Can you work these out from the model? Positions are in its coordinate system, mm. A direction names the side the tool comes from. Round coordinates to 2 decimals unless told otherwise and drop trailing zeros. Order: outer loops, then holes, each group sorted by start corner. A loop starts at its lowest first (then second) coordinate and runs counter-clockwise, first axis right, second up. Notation, with made-up numbers: (62.5, 50) -> (85.5, 50) arc R14 ccw to (85.5, 59) -> close; hole circle Ø9 at (-24, 54). An arc over 180 degrees is marked (long way). One line per item, written item: value.
```python
from build123d import *

# Parameters (mm, degrees)
EXTRUDE001_DEPTH = 3
EXTRUDE_DEPTH    = 5
PAD_DEPTH        = 6


with BuildPart() as extrude001:
    # RegularPolygon001 → Extrude001 (new body)
    with BuildSketch(Plane(origin=(0, 0, -2), x_dir=(0, 1, 0), z_dir=(0, 0, 1))):
        Polygon((0, -2.31), (2.000519, -1.155), (2.000519, 1.155), (0, 2.31), (-2.000519, 1.155), (-2.000519, -1.155), align=None)
    extrude(amount=-EXTRUDE001_DEPTH)


with BuildPart() as extrude_body:
    # RegularPolygon → Extrude (new body)
    with BuildSketch(Plane(origin=(0, 0, 0), x_dir=(0, 1, 0), z_dir=(0, 0, 1))):
        Polygon((0, -4.85), (4.200223, -2.425), (4.200223, 2.425), (0, 4.85), (-4.200223, 2.425), (-4.200223, -2.425), align=None)
    extrude(amount=-EXTRUDE_DEPTH)


with BuildPart() as fusion:
    # Sketch → Pad (new body)
    with BuildSketch(Plane.XY):
        with BuildLine():
            ThreePointArc((1.737208, 7.038793), (0, 9), (-1.737208, 7.038793))
            ThreePointArc((-3.748787, 6.20557), (-2.356657, 5.689474), (-1.737208, 7.038793))
            ThreePointArc((-3.748787, 6.20557), (-6.363961, 6.363961), (-6.20557, 3.748787))
            ThreePointArc((-7.038793, 1.737208), (-5.689474, 2.356657), (-6.20557, 3.748787))
            ThreePointArc((-7.038793, 1.737208), (-9, 0), (-7.038793, -1.737208))
            ThreePointArc((-6.20557, -3.748787), (-5.689474, -2.356657), (-7.038793, -1.737208))
            ThreePointArc((-6.20557, -3.748787), (-6.363961, -6.363961), (-3.748787, -6.20557))
            ThreePointArc((-1.737208, -7.038793), (-2.356657, -5.689474), (-3.748787, -6.20557))
            ThreePointArc((-1.737208, -7.038793), (0, -9), (1.737208, -7.038793))
            ThreePointArc((3.748787, -6.20557), (2.356657, -5.689474), (1.737208, -7.038793))
            ThreePointArc((3.748787, -6.20557), (6.363961, -6.363961), (6.20557, -3.748787))
            ThreePointArc((7.038793, -1.737208), (5.689474, -2.356657), (6.20557, -3.748787))
            ThreePointArc((7.038793, -1.737208), (9, 0), (7.038793, 1.737208))
            ThreePointArc((6.20557, 3.748787), (5.689474, 2.356657), (7.038793, 1.737208))
            ThreePointArc((6.20557, 3.748787), (6.363961, 6.363961), (3.748787, 6.20557))
            ThreePointArc((1.737208, 7.038793), (2.356657, 5.689474), (3.748787, 6.20557))
        make_face()
    extrude(amount=-PAD_DEPTH)

    # Cut: cut Extrude body
    add(extrude_body.part, mode=Mode.SUBTRACT)

    # Fusion: union Extrude001
    add(extrude001.part)


solid = fusion.part
```
Q1. Will these pins go through, and if not, where does the flat tip stop? pin 1 Ø2 at (y, z) = (-1.5, -4) entering from -X; pin 2 Ø6.5 at (x, y) = (-1.5, -1.5) entering from +Z; pin 3 Ø3 at (x, y) = (1, 0.5) entering from +Z; pin 4 Ø1.5 at (x, z) = (1, -2) entering from -Y.
Answers below:
pin 1: x = -8.93
pin 2: z = 0
pin 3: z = -2
pin 4: y = -8.98
Q2. I want a section at D-D on z = -5.45. List the corners of the cut face in (x, y) for me, plus the area to 3 significant figures.
Answers below:
outline: (-7.04, -1.74) arc R1.09 cw to (-6.21, -3.75) arc R1.75 ccw (long way) to (-3.75, -6.21) arc R1.09 cw to (-1.74, -7.04) arc R1.75 ccw (long way) to (1.74, -7.04) arc R1.09 cw to (3.75, -6.21) arc R1.75 ccw (long way) to (6.21, -3.75) arc R1.09 cw to (7.04, -1.74) arc R1.75 ccw (long way) to (7.04, 1.74) arc R1.09 cw to (6.21, 3.75) arc R1.75 ccw (long way) to (3.75, 6.21) arc R1.09 cw to (1.74, 7.04) arc R1.75 ccw (long way) to (-1.74, 7.04) arc R1.09 cw to (-3.75, 6.21) arc R1.75 ccw (long way) to (-6.21, 3.75) arc R1.09 cw to (-7.04, 1.74) arc R1.75 ccw (long way) to start
area: 191 mm^2
Q3. We'd pull the mould along Y, two halves only. Please class faces 3 (the face through (4, -2, 0)), 4 (the face through (0, -4.2, -2)): released by +Y, released by -Y, zero draft, split by the parting line, or undercut.
Answers below:
face 3: zero draft
face 4: undercut
Q4. I want a section at A-A on x = 0. List the corners of the cut face in (y, z) for me, plus the area to 3 significant figures.
Answers below:
outline: (-9, -6) -> (9, -6) -> (9, 0) -> (4.2, 0) -> (4.2, -5) -> (2, -5) -> (2, -2) -> (-2, -2) -> (-2, -5) -> (-4.2, -5) -> (-4.2, 0) -> (-9, 0) -> close
area: 78.0 mm^2
Q5. On a 3-axis mill with a long thin cutter (end or side, diameter ignored), from which of +Z, -Z, +X, -X, +Y, -Y can I reach the whole of each face in a straight line? I mean faces 1 (the face through (1.74, 0.99, -3.48)), 2 (the face through (5.698, -2.336, -2.958)). Say none if no direction works.
Answers below:
face 1: +Z
face 2: +Z, -Z
Q6. Please list where these lines run through material, in increasing order: line 1 along X through (y, z) = (1.25, -4.5); line 2 along Y through (x, z) = (-1, -4.95); line 3 along Y through (x, z) = (0.5, -4.6).
Answers below:
line 1: -8.47 to -4.13, -1.59 to 1.59, 4.13 to 8.47
line 2: -8.69 to -4.2, -2 to 2, 4.2 to 8.69
line 3: -8.93 to -4.2, -2 to 2, 4.2 to 8.93
Q7. I want a section at B-B on z = -4.1. List the corners of the cut face in (x, y) for me (3 decimals), plus the area to 3 significant figures.
Answers below:
outline: (-7.039, -1.737) arc R1.092 cw to (-6.206, -3.749) arc R1.75 ccw (long way) to (-3.749, -6.206) arc R1.092 cw to (-1.737, -7.039) arc R1.75 ccw (long way) to (1.737, -7.039) arc R1.092 cw to (3.749, -6.206) arc R1.75 ccw (long way) to (6.206, -3.749) arc R1.092 cw to (7.039, -1.737) arc R1.75 ccw (long way) to (7.039, 1.737) arc R1.092 cw to (6.206, 3.749) arc R1.75 ccw (long way) to (3.749, 6.206) arc R1.092 cw to (1.737, 7.039) arc R1.75 ccw (long way) to (-1.737, 7.039) arc R1.092 cw to (-3.749, 6.206) arc R1.75 ccw (long way) to (-6.206, 3.749) arc R1.092 cw to (-7.039, 1.737) arc R1.75 ccw (long way) to start; (-2.31, 0) -> (-1.155, -2.001) -> (1.155, -2.001) -> (2.31, 0) -> (1.155, 2.001) -> (-1.155, 2.001) -> close; hole (-4.85, 0) -> (-2.425, -4.2) -> (2.425, -4.2) -> (4.85, 0) -> (2.425, 4.2) -> (-2.425, 4.2) -> close
area: 144 mm^2
Q8. I want a section at C-C on y = 6.5. List the corners of the cut face in (x, z) for me, plus the area to 3 significant figures.
Answers below:
outline: (-6.21, -6) -> (-4.04, -6) -> (-4.04, 0) -> (-6.21, 0) -> close; (-1.7, -6) -> (1.7, -6) -> (1.7, 0) -> (-1.7, 0) -> close; (4.04, -6) -> (6.21, -6) -> (6.21, 0) -> (4.04, 0) -> close
area: 46.4 mm^2
